```python
from build123d import *

# Parameters (mm, degrees)
SKETCH1_R           = 10
SKETCH1_R_2         = 1.75
BOSS_EXTRUDE1_DEPTH = 7
SKETCH2_R           = 1.5
BOSS_EXTRUDE2_DEPTH = 5


with BuildPart() as part:
    # Sketch1 → Boss-Extrude1 (new body)
    with BuildSketch(Plane(origin=(0, 0, 0), x_dir=(1, 0, 0), z_dir=(0, 1, 0))):
        Circle(SKETCH1_R)
        with Locations((0, 5.5)):
            Circle(SKETCH1_R_2, mode=Mode.SUBTRACT)
        with Locations((5.5, 0)):
            Circle(SKETCH1_R_2, mode=Mode.SUBTRACT)
        with Locations((0, -5.5)):
            Circle(SKETCH1_R_2, mode=Mode.SUBTRACT)
        with Locations((-5.5, 0)):
            Circle(SKETCH1_R_2, mode=Mode.SUBTRACT)
    extrude(amount=BOSS_EXTRUDE1_DEPTH)

    # Sketch2 → Boss-Extrude2 (add)
    with BuildSketch(Plane(origin=(0, 7, 0), x_dir=(1, 0, 0), z_dir=(0, 1, 0))):
        with BuildLine():
            Line((2, 9.797958971), (30.8, 3.919183588))
            ThreePointArc((30.8, 3.919183588), (34, 0), (30.8, -3.919183588))
            Line((30.8, -3.919183588), (2, -9.797958971))
            ThreePointArc((2, -9.797958971), (10, 0), (2, 9.797958971))
        make_face()
        with Locations((30, 0)):
            Circle(SKETCH2_R, mode=Mode.SUBTRACT)
    extrude(amount=-BOSS_EXTRUDE2_DEPTH)


solid = part.part
```
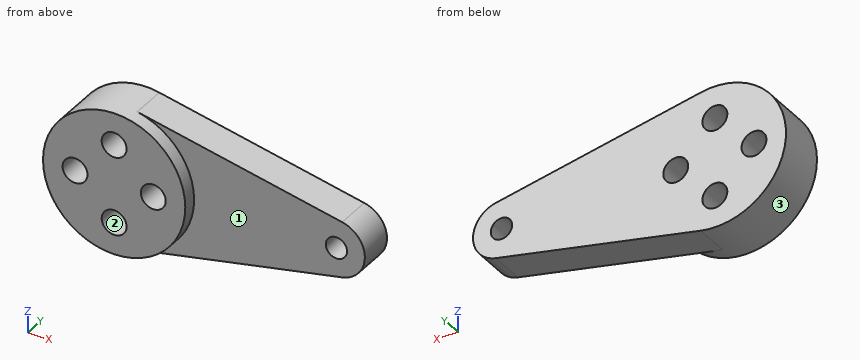
The listing builds one solid part. Answer for the finished solid, in the listing's coordinates (mm). Face numbers are marked on the shaded views. Coordinates: 2 decimals unless noted, no trailing zeros. Write each loop counter-clockwise with the first axis right and the second up, starting at its lowest first coordinate (ties: lowest second). Pieces come first, ordered by that corner, then holes. Notation, with made-up numbers: M 30.5,71.5 L 68.5,71.5 A35 cw 68.5,104.5 Z; hole C 81.25,28.5 d2. An arc over 180 degrees is marked long. Use a Markdown table: item, result. Add a question column.
1. For a pull along Z with two mould halves and no side action, classify the marked faces 1, 2 and 3 as +Z half, -Z half, draft (parallel to the pull), parting line (faces both ways), or undercut.
2. Section D-D (x = 5.5) is taken. Give the vertices of the cut face in (y, z), plus the area to 3 significant figures.
3. Section C-C (y = 3.75) is taken. Give the vertices of the cut face in (x, z), plus the area to 3 significant figures.
4. Straight lines are drawn through the part: line 1 along X through (y, z) = (3.8, 0); line 2 along Z through (x, y) = (0, 5.75); line 3 along Y through (x, z) = (18.5, -1.25). For each, find the intervals that lie inside material, in ascending order. Write a range as [from, to].
5. Section B-B (x = 0) is taken. Give the vertices of the cut face in (y, z).
6. Given P1, Ø2, axis at x = -5.5, z = 0, coming from the -Y side; P2, Ø4, axis at y = 5, z = 5, coming from the -X side; P3, Ø5, axis at x = 30, z = 0, coming from the -Y side; P4, Ø4, axis at y = 3, z = 4, coming from the +X side, each flat-ended and moving along its own axis, determine where each tip first touches the part or whether it passes through.
7. Section A-A (z = 0) is taken. Give the vertices of the cut face in (x, y), plus the area to 3 significant figures.
Data:
| question | item | result |
|---|---|---|
| 1 | face 1 | draft |
| 1 | face 2 | undercut |
| 1 | face 3 | parting line |
| 2 | outline | M 0,-8.35 L 2,-8.35 L 2,-9.08 L 7,-9.08 L 7,-1.75 L 0,-1.75 Z; M 0,1.75 L 7,1.75 L 7,9.08 L 2,9.08 L 2,8.35 L 0,8.35 Z |
| 2 | area | 99.7 mm2 |
| 3 | outline | M 2,-9.8 L 30.8,-3.92 A4 ccw 30.8,3.92 L 2,9.8 A10 ccw long Z; hole C -5.5,0 d3.5; hole C 0,-5.5 d3.5; hole C 0,5.5 d3.5; hole C 5.5,0 d3.5; hole C 30,0 d3 |
| 3 | area | 565 mm2 |
| 4 | line 1 | x = [-10, -7.25], [-3.75, 3.75], [7.25, 28.5], [31.5, 34] |
| 4 | line 2 | z = [-10, -7.25], [-3.75, 3.75], [7.25, 10] |
| 4 | line 3 | y = [2, 7] |
| 5 | outline | M 0,-10 L 7,-10 L 7,-7.25 L 0,-7.25 Z; M 0,-3.75 L 7,-3.75 L 7,3.75 L 0,3.75 Z; M 0,7.25 L 7,7.25 L 7,10 L 0,10 Z |
| 6 | P1 | passes through |
| 6 | P2 | stops at x = -9.54 |
| 6 | P3 | stops at y = 2 |
| 6 | P4 | stops at x = 33.46 |
| 7 | outline | M -10,0 L -7.25,0 L -7.25,7 L -10,7 Z; M -3.75,0 L 3.75,0 L 3.75,7 L -3.75,7 Z; M 7.25,0 L 10,0 L 10,2 L 28.5,2 L 28.5,7 L 7.25,7 Z; M 31.5,2 L 34,2 L 34,7 L 31.5,7 Z |
| 7 | area | 196 mm2 |
